Model file for the job. Use its own axes, mm. Round coordinates to 2 decimals unless told otherwise and drop trailing zeros. Loops run counter-clockwise (first coordinate to the right, second up) from the corner with the lowest first, then second, coordinate; pieces in that order, holes last. Notation, with made-up numbers: M -26.75,82 L 3.25,82 A21 cw 3.25,99 Z; hole C 11,33 d1. An arc over 180 degrees is marked long. Use a Markdown table: item, result. Add a question column.
Item 1: Saw through at B-B on y = 0.75. Write the cut outline in (x, z), then the cut area to 3 significant figures.
Item 2: Wall check: L1, parallel to Y at x = -29, z = -2.5 (3 decimals); L2, parallel to X at y = 0.5, z = -5; L3, parallel to X at y = -0.25, z = -8.75. Give the ranges that are in metal, low to high. Write a range as from..to.
Item 3: Pin check, flat tip, straight feed: P1, Ø3, axis at y = -2, z = 5, coming from the -X side. Stop position of the tip, or through.
```python
from build123d import *

# Parameters (mm, degrees)
SKETCH1_W           = 76.2
SKETCH1_H           = 25.4
BOSS_EXTRUDE1_DEPTH = 3.175
CHAMFER8_SIZE2      = 10.998522628
CHAMFER8_SIZE       = 6.35


with BuildPart() as part:
    # Sketch1 → Boss-Extrude1 (new, symmetric)
    with BuildSketch(Plane(origin=(0, 0, 0), x_dir=(1, 0, 0), z_dir=(0, 1, 0))):
        Rectangle(SKETCH1_W, SKETCH1_H)
    extrude(amount=BOSS_EXTRUDE1_DEPTH, both=True)

    # Chamfer8
    chamfer8_edges = [part.edges().sort_by_distance(p)[0] for p in [
        (-38.1, 3.175, 0),
    ]]
    chamfer8_side = [part.faces().sort_by_distance(p)[0] for p in [
        (-38.1, 3.048, 0),
    ]]
    chamfer(chamfer8_edges, length=CHAMFER8_SIZE - 0.0001, length2=CHAMFER8_SIZE2 - 0.0001, reference=chamfer8_side[0])  # a hair under: the kernel refuses the full size


solid = part.part
```
Entries:
| question | item | result |
|---|---|---|
| 1 | outline | M -31.3,-12.7 L 38.1,-12.7 L 38.1,12.7 L -31.3,12.7 Z |
| 1 | area | 1,760 mm2 |
| 2 | L1 | -3.175..2.079 |
| 2 | L2 | -31.73..38.1 |
| 2 | L3 | -33.03..38.1 |
| 3 | P1 | x = -38.1 |
